The model under review builds one solid part; all positions refer to its coordinate system, in mm. Face numbers are marked on the shaded views. A direction names the side the tool comes from. Coordinates: 2 decimals unless noted, no trailing zeros. Order: outer loops, then holes, each group sorted by start corner. A loop starts at its lowest first (then second) coordinate and runs counter-clockwise, first axis right, second up.
```python
from build123d import *

# Parameters (mm, degrees)
SKETCH1_W            = 25
SKETCH1_H            = 18
BOSS_EXTRUDE1_DEPTH  = 20
SKETCH2_W            = 13
SKETCH2_H            = 20
CUT_EXTRUDE1_DEPTH   = 12
SKETCH5_W            = 5
SKETCH5_H            = 10
CUT_EXTRUDE4_DEPTH   = 8
SKETCH3_R            = 1.475
CUT_EXTRUDE2_DEPTH   = 10
LPATTERN1_COUNT      = 3
LPATTERN1_PITCH      = 5
LPATTERN1_COUNT_DIR2 = 4
LPATTERN1_PITCH_DIR2 = 5
CUT_EXTRUDE3_REACH   = 31.669
SKETCH4_W            = 5
SKETCH4_H            = 5
CHAMFER1_SIZE        = 2


with BuildPart() as part:
    # Sketch1 → Boss-Extrude1 (new body)
    with BuildSketch(Plane(origin=(0, 0, 0), x_dir=(0, 1, 0), z_dir=(0, 0, 1))):
        Rectangle(SKETCH1_W, SKETCH1_H)
    extrude(amount=BOSS_EXTRUDE1_DEPTH)

    # Sketch2 → Cut-Extrude1 (cut)
    with BuildSketch(Plane.XY.offset(20)):
        Rectangle(SKETCH2_W, SKETCH2_H)
    extrude(amount=-CUT_EXTRUDE1_DEPTH, mode=Mode.SUBTRACT)

    # Sketch5 → Cut-Extrude4 (cut)
    with BuildSketch(Plane.XY.offset(8)):
        with Locations((0, 5)):
            Rectangle(SKETCH5_W, SKETCH5_H)
    extrude(amount=-CUT_EXTRUDE4_DEPTH, mode=Mode.SUBTRACT)

    # Sketch3 → Cut-Extrude2 (cut)
    with BuildSketch(Plane(origin=(0, 0, 0), x_dir=(1, 0, 0), z_dir=(0, 0, -1))):
        with Locations(Location((-5, 7.5, 0), (0, 0, 180))):
            Circle(SKETCH3_R)
    cut_extrude2 = extrude(amount=-CUT_EXTRUDE2_DEPTH, mode=Mode.SUBTRACT)

    # LPattern1: Cut-Extrude2 3 × 4, 2 skipped
    with Locations(*[(i * LPATTERN1_PITCH, j * LPATTERN1_PITCH_DIR2, 0) for i in range(LPATTERN1_COUNT) for j in range(LPATTERN1_COUNT_DIR2) if (i, j) not in ((0, 0), (1, 2), (1, 3))]):
        add(cut_extrude2, mode=Mode.SUBTRACT)

    # Cut-Extrude3: up to this face of the body (flat: up to its plane)
    cut_extrude3_end = Plane(part.part.faces().sort_by_distance((2.5, 5, 4))[0])
    # Sketch4 → Cut-Extrude3 (cut, up to the picked face)
    with BuildSketch(Plane.YZ.offset(9), mode=Mode.PRIVATE) as cut_extrude3_sk1:
        with Locations((2.5, 5.5)):
            Rectangle(SKETCH4_W, SKETCH4_H)
    cut_extrude3_tool1 = split(extrude(cut_extrude3_sk1.sketch, amount=-CUT_EXTRUDE3_REACH, mode=Mode.PRIVATE), bisect_by=cut_extrude3_end, keep=Keep.BOTH, mode=Mode.PRIVATE)
    add(cut_extrude3_tool1.solids().sort_by(Axis((9, 2.5, 5.5), (-1, 0, 0)))[0], mode=Mode.SUBTRACT)

    # Chamfer1
    chamfer1_edges = [part.edges().sort_by_distance(p)[0] for p in [
        (2.5, 5, 5.5),
    ]]
    chamfer(chamfer1_edges, length=CHAMFER1_SIZE)


solid = part.part
```
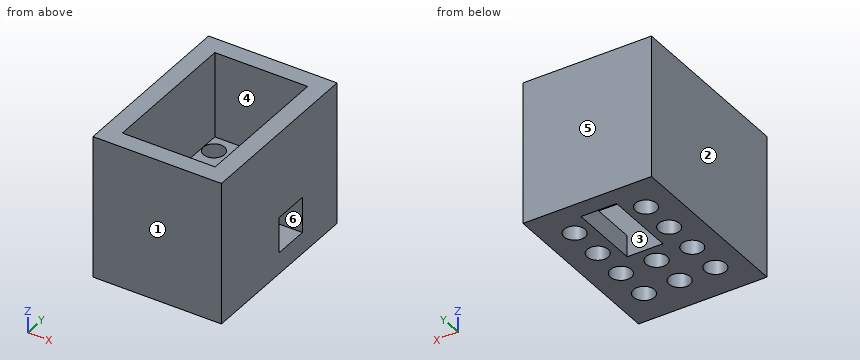
(1) Wall thickness on probe 1 along Y at (x, z) = (5, 1.7) (3 decimals); probe 2 along Y at (x, z) = (0, 4.5) (3 decimals); probe 3 along Y at (x, z) = (5, 5.5) (3 decimals): over which ranges is each line inside the solid? List them lowest first.
A:
probe 1: y = -12.5 to -8.975, -6.025 to -3.975, -1.025 to 1.025, 3.975 to 6.025, 8.975 to 12.5
probe 2: y = -12.5 to -8.975, -6.025 to -3.975, -1.025 to 0, 10 to 12.5
probe 3: y = -12.5 to -8.975, -6.025 to -3.975, -1.025 to 0, 5 to 6.025, 8.975 to 12.5
(2) We need section C-C, the plane y = 4.5. Write out the cut boundary in (x, z).
A:
outline: (-9, 0) - (-2.5, 0) - (-2.5, 8) - (-6.5, 8) - (-6.5, 20) - (-9, 20) - close; (2.5, 0) - (9, 0) - (9, 3) - (2.5, 3) - close; (6.5, 8) - (9, 8) - (9, 20) - (6.5, 20) - close
(3) We need section D-D, the plane z = 6. Count the separate pieces of the cut face and the enclosed holes in it, and give its area (3 significant figures).
A:
separate pieces: 1
enclosed holes: 9
area: 304 mm2
(4) Machinability: for the marked faces 4, 5 and 6, which of the approach directions +Z, -Z, +X, -X, +Y, -Y give a long, thin tool a straight path to every point of the face, cutting with its end or side? Answer none if there is none.
A:
face 4: +Z
face 5: +Z, -Z, +X, -X, +Y
face 6: +X
(5) For pin 1 Ø4 at (x, y) = (0, -7.5) entering from +Z, flat-tipped, find the tip position at first contact; note if it passes through.
A:
pin 1: stops at z = 8
(6) We need section B-B, the plane x = 0. Write out the cut boundary in (y, z) (3 decimals), and give its area (3 significant figures).
A:
outline: (-12.5, 0) - (-8.975, 0) - (-8.975, 8) - (-10, 8) - (-10, 20) - (-12.5, 20) - close; (-6.025, 0) - (-3.975, 0) - (-3.975, 8) - (-6.025, 8) - close; (-1.025, 0) - (0, 0) - (0, 8) - (-1.025, 8) - close; (10, 0) - (12.5, 0) - (12.5, 20) - (10, 20) - close
area: 133 mm2
(7) We need section A-A, the plane y = 7.5. Write out the cut boundary in (x, z) (3 decimals), and give its area (3 significant figures).
A:
outline: (-9, 0) - (-6.475, 0) - (-6.475, 8) - (-6.5, 8) - (-6.5, 20) - (-9, 20) - close; (-3.525, 0) - (-2.5, 0) - (-2.5, 8) - (-3.525, 8) - close; (2.5, 0) - (3.525, 0) - (3.525, 8) - (2.5, 8) - close; (6.475, 0) - (9, 0) - (9, 20) - (6.5, 20) - (6.5, 8) - (6.475, 8) - close
area: 117 mm2
(8) Draft analysis for pull direction Y (two halves, no side actions). For the marked faces 1, 2 and 3, state which applies: released by +Y, released by -Y, zero draft, split by the parting line, or undercut.
A:
face 1: released by -Y
face 2: zero draft
face 3: undercut
